Input: part model. Units: mm. Frame: model coordinates. A direction names the side the tool comes from. Give positions to 0.01 mm unless a question says otherwise; leave off trailing zeros. Loops run counter-clockwise (first coordinate to the right, second up) from the corner with the lowest first, then second, coordinate; pieces in that order, holes last. Notation, with made-up numbers: (66.25, 18.25) -> (74.25, 18.25) arc R19 ccw to (74.25, 29.25) -> close; hole circle Ø3 at (78.25, 62.25). An arc over 180 degrees is marked (long way). Answer as a JSON object with one key per item and string values.
```python
from build123d import *

# Parameters (mm, degrees)
SKETCH_W           = 7
SKETCH_H           = 7
PAD_DEPTH          = 1.58
POCKET_DEPTH       = 0.5
SKETCH002_W        = 1.02
SKETCH002_H        = 1.02
PAD001_DEPTH       = 2.66
POLARPATTERN_COUNT = 4
SKETCH003_R        = 2.03
POCKET001_DEPTH    = 0.2
SKETCH004_R        = 0.635
PAD002_DEPTH       = 3.36
CHAMFER_SIZE       = 0.2
CHAMFER001_SIZE    = 0.1
CHAMFER002_SIZE    = 0.1


with BuildPart() as part:
    # Sketch → Pad (new body)
    with BuildSketch(Plane.XY):
        Rectangle(SKETCH_W, SKETCH_H)
    extrude(amount=PAD_DEPTH)

    # Sketch001 (on Face5 of Pad) → Pocket (cut)
    with BuildSketch(Plane(origin=(0, 0, 0), x_dir=(1, 0, 0), z_dir=(0, 0, -1))):
        Polygon((-3.5, 2.03), (-2.03, 2.03), (-2.03, 3.5), (2.03, 3.5), (2.03, 2.03), (3.5, 2.03), (3.5, -2.03), (2.03, -2.03), (2.03, -3.5), (-2.03, -3.5), (-2.03, -2.03), (-3.5, -2.03), align=None)
    extrude(amount=-POCKET_DEPTH, mode=Mode.SUBTRACT)

    # Sketch002 (on Face6 of Pocket) → Pad001 (join)
    with BuildSketch(Plane(origin=(0, 0, 0), x_dir=(1, 0, 0), z_dir=(0, 0, -1))):
        with Locations((-2.54, 2.54)):
            Rectangle(SKETCH002_W, SKETCH002_H)
    pad001 = extrude(amount=PAD001_DEPTH)

    # PolarPattern: Pad001 ×4 about axis
    polarpattern_axis = Axis((0, 0, 0), (0, 0, -1))
    for i in range(1, POLARPATTERN_COUNT):
        add(pad001.rotate(polarpattern_axis, i * 360 / POLARPATTERN_COUNT))

    # Sketch003 (on Face4 of PolarPattern) → Pocket001 (cut)
    with BuildSketch(Plane(origin=(0, 0, 0.5), x_dir=(1, 0, 0), z_dir=(0, 0, -1))):
        Circle(SKETCH003_R)
    extrude(amount=-POCKET001_DEPTH, mode=Mode.SUBTRACT)

    # Sketch004 (on Face33 of Pocket001) → Pad002 (join)
    with BuildSketch(Plane(origin=(0, 0, 0.7), x_dir=(1, 0, 0), z_dir=(0, 0, -1))):
        Circle(SKETCH004_R)
    extrude(amount=PAD002_DEPTH)

    # Chamfer
    chamfer_edges = [part.edges().sort_by_distance(p)[0] for p in [
        (-0.635, 0, -2.66),
    ]]
    chamfer(chamfer_edges, length=CHAMFER_SIZE)

    # Sketch005 → Revolution (revolve)
    with BuildSketch(Plane.XZ):
        Polygon((0, 1.58), (0, 12.26), (0.48, 12.26), (0.48, 15.46), (0.63, 15.46), (0.63, 14.96), (1.9, 14.96), (1.9, 15.58), (2.325, 15.58), (2.325, 17.58), (2.65, 17.58), (2.65, 2.766921), (3.095, 2.51), (3.095, 1.58), align=None)
    revolve(axis=Axis((0, 0, 0), (0, 0, 1)))

    # Chamfer001
    chamfer001_edges = [part.edges().sort_by_distance(p)[0] for p in [
        (-2.325, 0, 17.58),
        (-2.65, 0, 17.58),
    ]]
    chamfer(chamfer001_edges, length=CHAMFER001_SIZE)

    # Chamfer002
    chamfer002_edges = [part.edges().sort_by_distance(p)[0] for p in [
        (-0.48, 0, 15.46),
    ]]
    chamfer(chamfer002_edges, length=CHAMFER002_SIZE)

    # Sketch006 → Revolution001 (revolve)
    with BuildSketch(Plane.XZ):
        Polygon((2.65, 2.791559), (3.095, 3.04848), (3.095, 3.21612), (2.65, 3.473041), align=None)
        Polygon((2.65, 3.497679), (3.095, 3.7546), (3.095, 3.92224), (2.65, 4.179161), align=None)
        Polygon((2.65, 4.203799), (3.095, 4.46072), (3.095, 4.62836), (2.65, 4.885281), align=None)
        Polygon((2.65, 4.909919), (3.095, 5.16684), (3.095, 5.33448), (2.65, 5.591401), align=None)
        Polygon((2.65, 5.616039), (3.095, 5.87296), (3.095, 6.0406), (2.65, 6.297521), align=None)
        Polygon((2.65, 6.322159), (3.095, 6.57908), (3.095, 6.74672), (2.65, 7.003641), align=None)
        Polygon((2.65, 7.734399), (3.095, 7.99132), (3.095, 8.15896), (2.65, 8.415881), align=None)
        Polygon((2.65, 7.028279), (3.095, 7.2852), (3.095, 7.45284), (2.65, 7.709761), align=None)
        Polygon((2.65, 8.440519), (3.095, 8.69744), (3.095, 8.86508), (2.65, 9.122001), align=None)
        Polygon((2.65, 9.146639), (3.095, 9.40356), (3.095, 9.5712), (2.65, 9.828121), align=None)
        Polygon((2.65, 10.558879), (3.095, 10.8158), (3.095, 10.98344), (2.65, 11.240361), align=None)
        Polygon((2.65, 9.852759), (3.095, 10.10968), (3.095, 10.27732), (2.65, 10.534241), align=None)
        Polygon((2.65, 11.971119), (3.095, 12.22804), (3.095, 12.39568), (2.65, 12.652601), align=None)
        Polygon((2.65, 11.264999), (3.095, 11.52192), (3.095, 11.68956), (2.65, 11.946481), align=None)
        Polygon((2.65, 12.677239), (3.095, 12.93416), (3.095, 13.1018), (2.65, 13.358721), align=None)
        Polygon((2.65, 13.383359), (3.095, 13.64028), (3.095, 13.80792), (2.65, 14.064841), align=None)
        Polygon((2.65, 14.089479), (3.095, 14.3464), (3.095, 14.51404), (2.65, 14.770961), align=None)
        Polygon((2.65, 15.501719), (3.095, 15.75864), (3.095, 15.92628), (2.65, 16.183201), align=None)
        Polygon((2.65, 16.207839), (3.095, 16.46476), (3.095, 16.6324), (2.65, 16.889321), align=None)
        Polygon((2.65, 14.795599), (3.095, 15.05252), (3.095, 15.22016), (2.65, 15.477081), align=None)
    revolve(axis=Axis((0, 0, 0), (0, 0, 1)))


solid = part.part
```
Q1. Access query for faces 4 (the cylindrical face through (0.46, 0.14, 13.83)), 5 (the flat face through (2.03, -2.6, -1.1)). Directions: +Z, -Z, +X, -X, +Y, -Y. A direction counts if a zero-diameter tool reaches every point of the face in a straight line with its end or side. Return the directions, or none.
Evaluation:
{"face 4": "+Z", "face 5": "-Z, +Y, -Y"}
Q2. Pin query (flat end, axial travel): pin 1 (1 mm diameter, centred on y = -2.5, z = 5.5, fed in from -X); pin 2 (2 mm diameter, centred on x = -0.5, y = 0, fed in from +Z); pin 3 (0.8 mm diameter, centred on x = 2.5, z = -2, fed in from +Y). Return the tip coordinate at first contact, or that it passes through.
Evaluation:
{"pin 1": "stops at x = -2.34", "pin 2": "stops at z = 15.46", "pin 3": "stops at y = 3.05"}
Q3. Section A-A, the plane z = -0.75. Return the cut outline in (x, y) (3 decimals).
Evaluation:
{"outline": "(-3.05, -3.05) -> (-2.03, -3.05) -> (-2.03, -2.03) -> (-3.05, -2.03) -> close; (-3.05, 2.03) -> (-2.03, 2.03) -> (-2.03, 3.05) -> (-3.05, 3.05) -> close; circle Ø1.27 at (0, 0); (2.03, -3.05) -> (3.05, -3.05) -> (3.05, -2.03) -> (2.03, -2.03) -> close; (2.03, 2.03) -> (3.05, 2.03) -> (3.05, 3.05) -> (2.03, 3.05) -> close"}
Q4. Ray query, line 1 along Y through (x, z) = (1, 13.25); line 2 along Z through (x, y) = (1.5, 0.5); line 3 along Z through (x, y) = (1, 2.25). Return the intervals inside material, ascending.
Evaluation:
{"line 1": "y = -2.66 to 2.66", "line 2": "z = 0.7 to 14.96", "line 3": "z = 0.5 to 17.58"}
Q5. Draft query along Y for faces 1 (the flat face through (-3.3, 2.9, 0)), 2 (the flat face through (2.6, 2.03, -1.1)), 3 (the flat face through (0, 3.5, 1)). Return one class per face: +Y half, -Y half, draft (parallel to the pull), parting line (faces both ways), or undercut.
Evaluation:
{"face 1": "draft", "face 2": "undercut", "face 3": "+Y half"}
